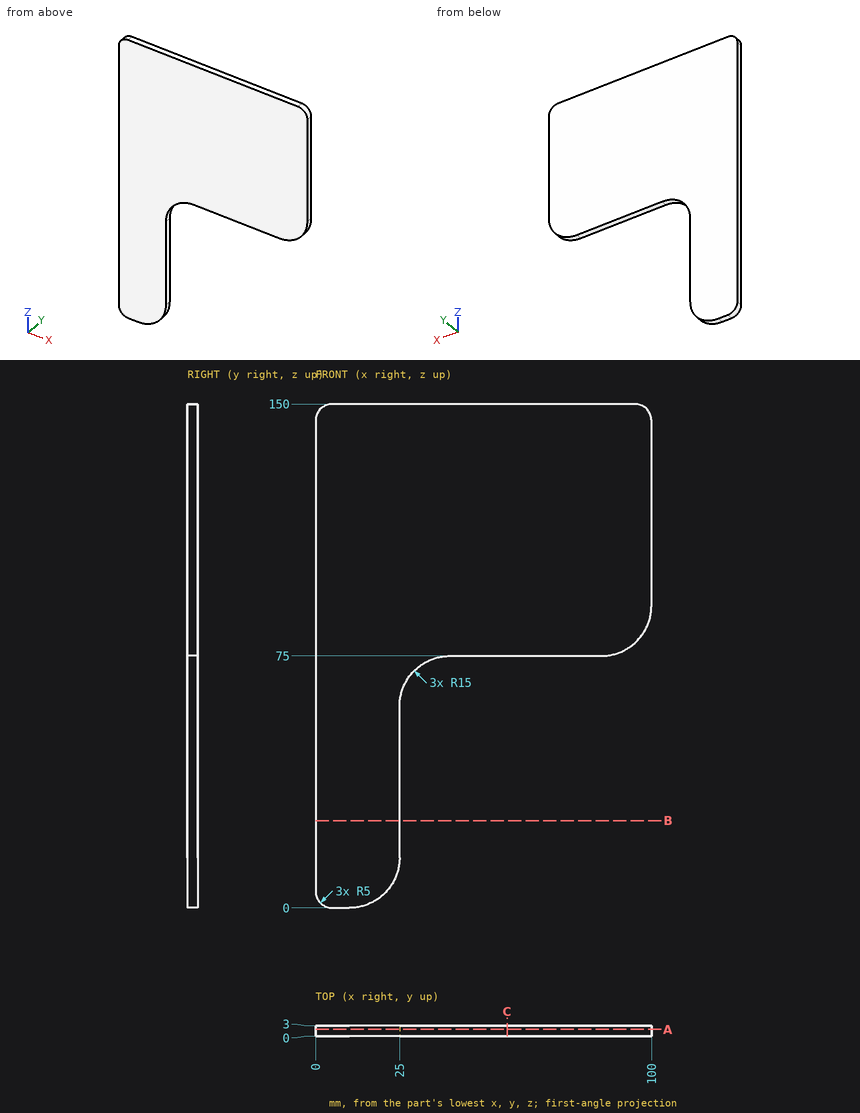
Here's the drawing with two shaded views (mm, measured from the low corner). I have some questions. Coordinates: 2 decimals unless noted, no trailing zeros. Loops run counter-clockwise (first coordinate to the right, second up) from the corner with the lowest first, then second, coordinate; pieces in that order, holes last.
Item 1: I'm going to push a flat-ended pin straight in: pin 1 (1.5 mm diameter, centred on y = 1, z = 49.5, fed in from +X). Where does the tip first touch, or does it pass through?
Answers below:
pin 1: stops at x = 25
Item 2: Please list where these lines run through material, in increasing order: L1, parallel to Z at x = 61, y = 0.9; L2, parallel to X at y = 2.15, z = 16; L3, parallel to Z at x = 23, y = 0.2.
Answers below:
L1: z = 75 to 150
L2: x = 0 to 25
L3: z = 7.52 to 150
Item 3: Suppose I cut it at B-B (z = 26). Please give me the cut outline in (x, y), then the cut area to 3 significant figures.
Answers below:
outline: (0, 0) - (25, 0) - (25, 3) - (0, 3) - close
area: 75.0 mm2
Item 4: Suppose I cut it at A-A (y = 1.95). Please give me the cut outline in (x, z).
Answers below:
outline: (0, 5) arc R5 ccw to (5, 0) - (10, 0) arc R15 ccw to (25, 15) - (25, 60) arc R15 cw to (40, 75) - (85, 75) arc R15 ccw to (100, 90) - (100, 145) arc R5 ccw to (95, 150) - (5, 150) arc R5 ccw to (0, 145) - close
Item 5: Suppose I cut it at C-C (x = 57). Please give me the cut outline in (y, z).
Answers below:
outline: (0, 75) - (3, 75) - (3, 150) - (0, 150) - close
